Print and shaded views of the part. All mm, measured from the part's lowest x, y and z. A direction names the side the tool comes from. Round coordinates to 2 decimals unless told otherwise and drop trailing zeros. Loops run counter-clockwise (first coordinate to the right, second up) from the corner with the lowest first, then second, coordinate; pieces in that order, holes last. Notation, with made-up numbers: (57, -7) -> (99, -7) arc R23 cw to (99, 27) -> close; hole circle Ø5 at (20, 29.5). An arc over 180 degrees is marked (long way). Use a Markdown table: item, result.
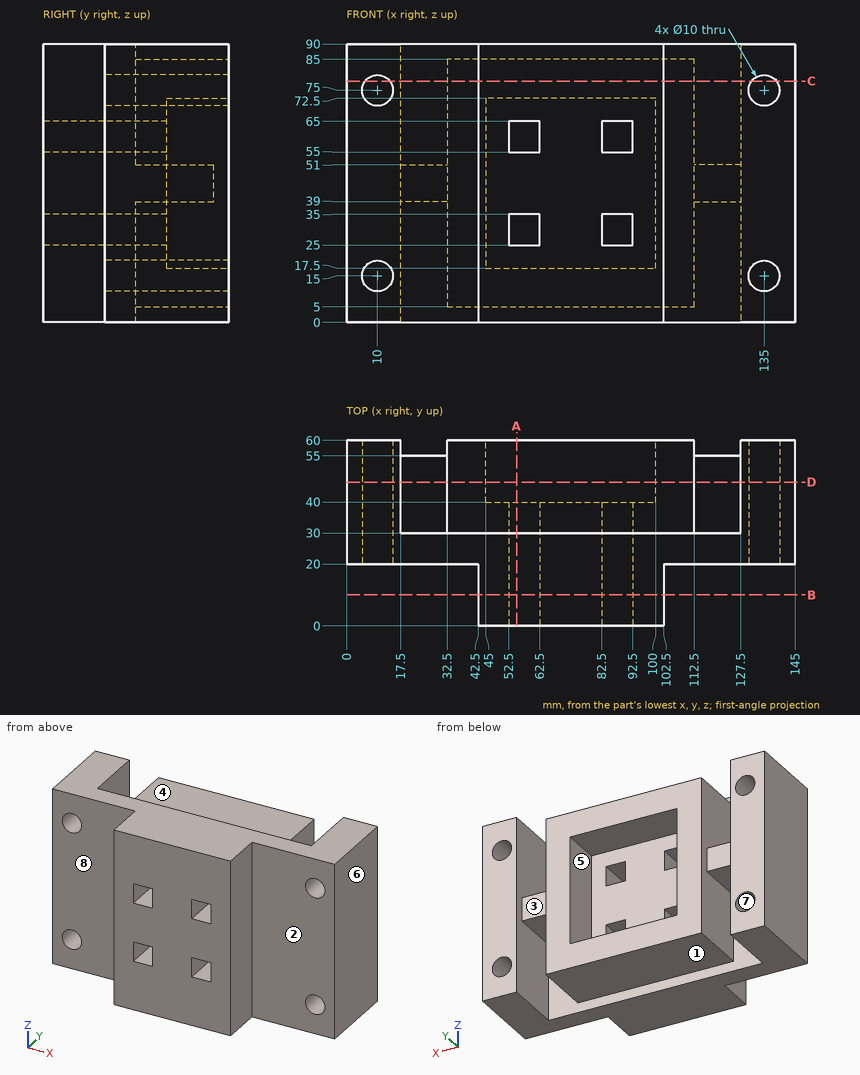
Q1. Flat gauge pins, fed straight in: pin 1 (10 mm diameter, centred on x = 95.5, z = 78.5, fed in from -Y); pin 2 (15 mm diameter, centred on x = 64, y = 40.5, fed in from -Z); pin 3 (4.5 mm diameter, centred on x = 118, y = 44, fed in from -Z); pin 4 (13 mm diameter, centred on x = 20.5, z = 47, fed in from -Y). Where does each tip first touch, or does it go through?
Results list:
| item | result |
|---|---|
| pin 1 | stops at y = 0 |
| pin 2 | stops at z = 5 |
| pin 3 | stops at z = 39 |
| pin 4 | stops at y = 20 |
Q2. Band-saw the part on B-B, the plane y = 10. Give the cut face in (x, z).
Results list:
| item | result |
|---|---|
| outline | (42.5, 0) -> (102.5, 0) -> (102.5, 90) -> (42.5, 90) -> close; hole (52.5, 25) -> (62.5, 25) -> (62.5, 35) -> (52.5, 35) -> close; hole (52.5, 55) -> (62.5, 55) -> (62.5, 65) -> (52.5, 65) -> close; hole (82.5, 25) -> (92.5, 25) -> (92.5, 35) -> (82.5, 35) -> close; hole (82.5, 55) -> (92.5, 55) -> (92.5, 65) -> (82.5, 65) -> close |
Q3. Tool access for the marked faces 1, 2, 3, 4 and 5: list every direction of +Z, -Z, +X, -X, +Y, -Y with a clear straight run to the whole face (end or side of a thin tool).
Results list:
| item | result |
|---|---|
| face 1 | -Z, +Y |
| face 2 | +Z, -Z, +X, -Y |
| face 3 | +Z, -Z, +Y |
| face 4 | +Z, +Y |
| face 5 | +Y |
Q4. Band-saw the part on C-C, the plane z = 78. Give the cut face in (x, y).
Results list:
| item | result |
|---|---|
| outline | (0, 20) -> (6, 20) -> (6, 60) -> (0, 60) -> close; (14, 20) -> (42.5, 20) -> (42.5, 0) -> (102.5, 0) -> (102.5, 20) -> (131, 20) -> (131, 60) -> (127.5, 60) -> (127.5, 30) -> (112.5, 30) -> (112.5, 60) -> (32.5, 60) -> (32.5, 30) -> (17.5, 30) -> (17.5, 60) -> (14, 60) -> close; (139, 20) -> (145, 20) -> (145, 60) -> (139, 60) -> close |
Q5. Drill centre lines: L1, parallel to Z at x = 10, y = 42; L2, parallel to X at y = 42, z = 57; L3, parallel to X at y = 23, z = 28.5. Where is each one in solid material? Low to high. Write a range as from..to.
Results list:
| item | result |
|---|---|
| L1 | z = 0..10, 20..70, 80..90 |
| L2 | x = 0..17.5, 32.5..45, 100..112.5, 127.5..145 |
| L3 | x = 0..52.5, 62.5..82.5, 92.5..145 |
Q6. Band-saw the part on D-D, the plane y = 46.5. Give the cut face in (x, z), plus the area to 3 significant figures.
Results list:
| item | result |
|---|---|
| outline | (0, 0) -> (17.5, 0) -> (17.5, 39) -> (32.5, 39) -> (32.5, 5) -> (112.5, 5) -> (112.5, 39) -> (127.5, 39) -> (127.5, 0) -> (145, 0) -> (145, 90) -> (127.5, 90) -> (127.5, 51) -> (112.5, 51) -> (112.5, 85) -> (32.5, 85) -> (32.5, 51) -> (17.5, 51) -> (17.5, 90) -> (0, 90) -> close; hole circle Ø10 at (10, 15); hole circle Ø10 at (10, 75); hole (45, 17.5) -> (100, 17.5) -> (100, 72.5) -> (45, 72.5) -> close; hole circle Ø10 at (135, 15); hole circle Ø10 at (135, 75) |
| area | 6,570 mm² |
Q7. Band-saw the part on A-A, the plane x = 55. Give the cut face in (y, z).
Results list:
| item | result |
|---|---|
| outline | (0, 0) -> (30, 0) -> (30, 5) -> (60, 5) -> (60, 17.5) -> (40, 17.5) -> (40, 25) -> (0, 25) -> close; (0, 35) -> (40, 35) -> (40, 55) -> (0, 55) -> close; (0, 65) -> (40, 65) -> (40, 72.5) -> (60, 72.5) -> (60, 85) -> (30, 85) -> (30, 90) -> (0, 90) -> close |
Q8. Pull direction X, two halves, no side cores. Call the marked faces 6, 7 and 8: released by +X, released by -X, zero draft, split by the parting line, or undercut.
Results list:
| item | result |
|---|---|
| face 6 | released by +X |
| face 7 | undercut |
| face 8 | zero draft |
